Answer from the drawing. Dimensions are ordinates in mm from the lowest x, y and z of the part. Give positions to 0.01 mm unless a question says otherwise; leave off trailing zeros. Order: outer loops, then holes, each group sorted by start corner. A loop starts at its lowest first (then second) coordinate and runs counter-clockwise, first axis right, second up.
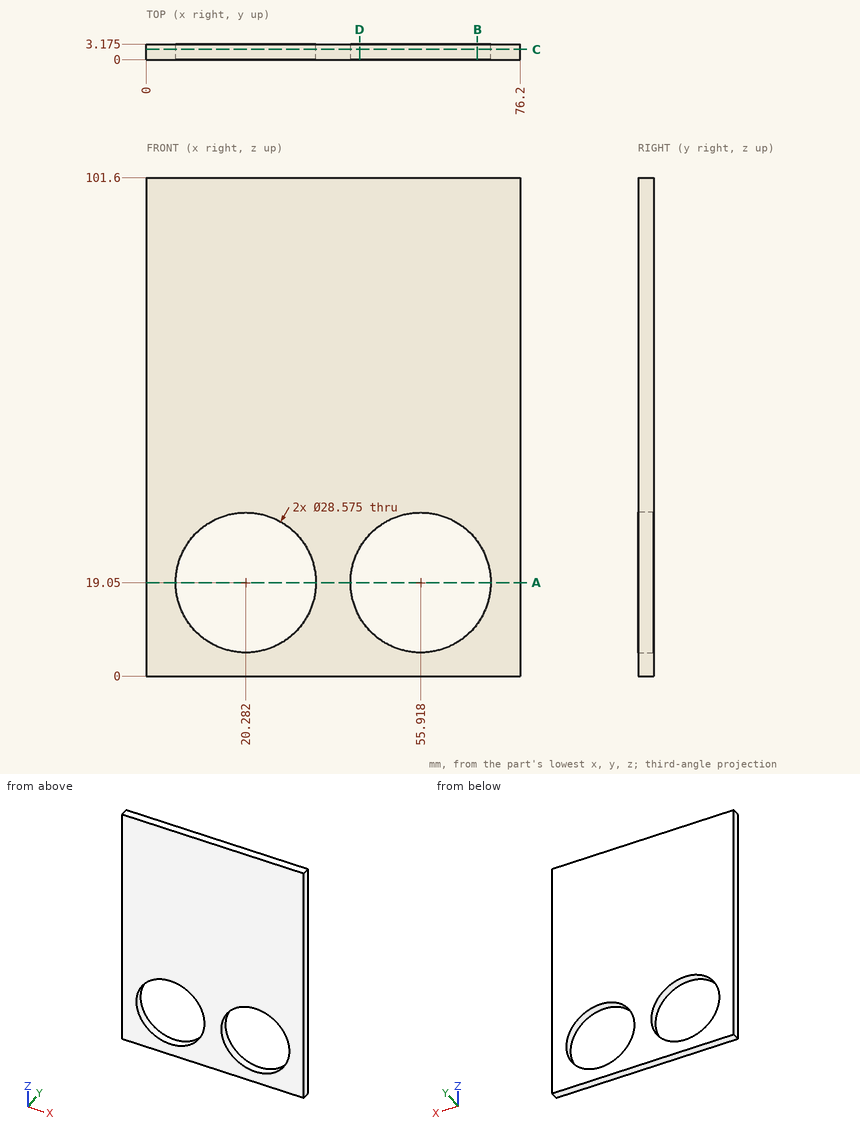
1. The part is cut by section A-A (z = 19.05). Write down the section's boundary in (x, y) (1 decimal), then the cut area to 3 significant figures.
Findings below:
outline: (0, 0) - (6, 0) - (6, 3.2) - (0, 3.2) - close; (34.6, 0) - (41.6, 0) - (41.6, 3.2) - (34.6, 3.2) - close; (70.2, 0) - (76.2, 0) - (76.2, 3.2) - (70.2, 3.2) - close
area: 60.5 mm2
2. The part is cut by section D-D (x = 43.5). Write down the section's boundary in (y, z) (1 decimal), then the cut area to 3 significant figures.
Findings below:
outline: (0, 0) - (3.2, 0) - (3.2, 12) - (0, 12) - close; (0, 26.1) - (3.2, 26.1) - (3.2, 101.6) - (0, 101.6) - close
area: 278 mm2
3. The part is cut by section B-B (x = 67.5). Write down the section's boundary in (y, z) (3 decimals).
Findings below:
outline: (0, 0) - (3.175, 0) - (3.175, 10.684) - (0, 10.684) - close; (0, 27.416) - (3.175, 27.416) - (3.175, 101.6) - (0, 101.6) - close
4. The part is cut by section C-C (y = 2.1). State how many separate pieces and enclosed holes the cut face has, then the cut area to 3 significant figures.
Findings below:
separate pieces: 1
enclosed holes: 2
area: 6,460 mm2
5. Straight lines are drawn through the part: probe 1 along X at (y, z) = (1.9, 19.05); probe 2 along Z at (x, y) = (20, 1.25); probe 3 along Z at (x, y) = (62, 2.8). For each, find the intervals that lie inside material, in ascending order.
Findings below:
probe 1: x = 0 to 5.99, 34.57 to 41.63, 70.21 to 76.2
probe 2: z = 0 to 4.77, 33.33 to 101.6
probe 3: z = 0 to 6.12, 31.98 to 101.6
